Here's how the part is built. I have some questions about the finished solid (model axes, mm). Face numbers are marked on the shaded views. A direction names the side the tool comes from. Give positions to 0.01 mm unless a question says otherwise; leave off trailing zeros. Write each loop counter-clockwise with the first axis right and the second up, starting at its lowest first coordinate (ties: lowest second). Pieces come first, ordered by that corner, then holes. Notation, with made-up numbers: (-23, -20.5) - (-1, -20.5) arc R22 cw to (-1, 14.5) - close; hole circle Ø10 at (52.25, -20). An arc over 180 degrees is marked (long way). Write each question's results on one line, items separated by ' | '. Start each with the question number.
Item 1: Suppose I cut it at C-C on x = -283.5. List the corners of the cut face in (y, z) for me.
Item 2: Suppose I cut it at B-B on z = 50.8. List the corners of the cut face in (x, y) for me.
Item 3: Will these pins go through, and if not, where does the flat tip stop? P1, Ø2, axis at y = 34.5, z = -12, coming from the -X side; P2, Ø3, axis at x = -248.5, y = 87.5, coming from the +Z side.
Item 4: We'd pull the mould along Y, two halves only. Please class the marked faces 1, 2 and 3: +Y half, -Y half, draft (parallel to the pull), parting line (faces both ways), or undercut.
Item 5: Which directions (+Z, -Z, +X, -X, +Y, -Y) give clear straight access to the entire face, cutting with the end or side of a thin tool? Please do the marked faces 4, 5 and 6.
Item 6: Suppose I cut it at D-D on x = -39. List the corners of the cut face in (y, z) for me.
Item 7: Suppose I cut it at A-A on y = 12.7. List the corners of the cut face in (x, z) for me.
Item 8: Please list where these lines run through material, in increasing order: line 1 along Z through (x, y) = (-79, 12); line 2 along Y through (x, z) = (-150.5, 50.8); line 3 along X through (y, z) = (-36, -40.5).
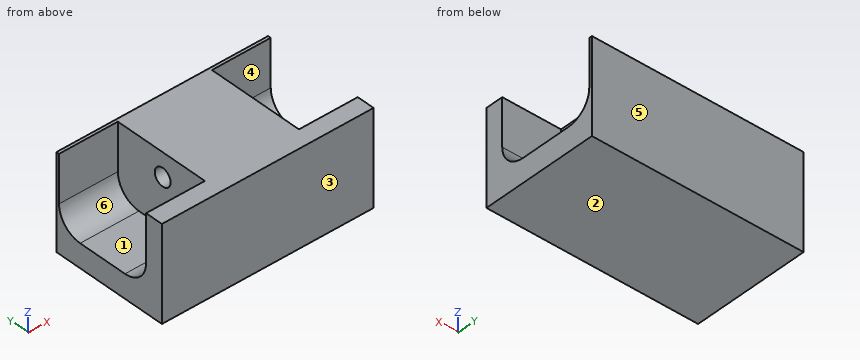
```python
from build123d import *

# Parameters (mm, degrees)
SKETCH1_W           = 203.2
SKETCH1_H           = 254
BOSS_EXTRUDE1_DEPTH = 114.3
CUT_EXTRUDE2_DEPTH  = 127
SKETCH3_R           = 19.05
CUT_EXTRUDE3_DEPTH  = 380.515441056


with BuildPart() as part:
    # Sketch1 → Boss-Extrude1 (new, symmetric)
    with BuildSketch(Plane(origin=(0, 0, 0), x_dir=(0, 0, -1), z_dir=(1, 0, 0))):
        Rectangle(SKETCH1_W, SKETCH1_H)
    extrude(amount=BOSS_EXTRUDE1_DEPTH, both=True)

    # Sketch2 → Cut-Extrude2 (cut)
    with BuildSketch(Plane(origin=(114.3, 0, 0), x_dir=(0, 0, -1), z_dir=(1, 0, 0))):
        with BuildLine():
            Line((-101.6, 120.65), (0, 120.65))
            ThreePointArc((0, 120.65), (35.921024484, 105.771024484), (50.8, 69.85))
            Line((50.8, 69.85), (50.8, -38.1))
            ThreePointArc((50.8, -38.1), (35.921024484, -74.021024484), (0, -88.9))
            Line((0, -88.9), (-101.6, -88.9))
            Line((-101.6, -88.9), (-101.6, 120.65))
        make_face()
    extrude(amount=-CUT_EXTRUDE2_DEPTH, mode=Mode.SUBTRACT)

    # Mirror1: part across plane


with BuildPart() as part_1:
    add(part.part)
    add(part.part.mirror(Plane(origin=(-114.3, 0, 0), x_dir=(0, 0, 1), z_dir=(1, 0, 0))))

    # Sketch3 → Cut-Extrude3 (cut, through all)
    with BuildSketch(Plane(origin=(0, 0, 0), x_dir=(0, 0, -1), z_dir=(1, 0, 0))):
        with Locations((-50.8, 12.7)):
            Circle(SKETCH3_R)
    extrude(amount=-CUT_EXTRUDE3_DEPTH, mode=Mode.SUBTRACT)


solid = part_1.part
```
Checked values:
1) outline: (-127, -101.6) - (127, -101.6) - (127, 101.6) - (120.65, 101.6) - (120.65, 0) arc R50.8 cw to (69.85, -50.8) - (-38.1, -50.8) arc R50.8 cw to (-88.9, 0) - (-88.9, 101.6) - (-127, 101.6) - close
2) outline: (-342.9, -127) - (114.3, -127) - (114.3, -88.9) - (-12.7, -88.9) - (-12.7, -6.35) - (-215.9, -6.35) - (-215.9, -88.9) - (-342.9, -88.9) - close; (-342.9, 120.65) - (-215.9, 120.65) - (-215.9, 31.75) - (-12.7, 31.75) - (-12.7, 120.65) - (114.3, 120.65) - (114.3, 127) - (-342.9, 127) - close
3) P1: stops at x = -215.9 | P2: stops at z = -47.05
4) face 1: undercut | face 2: draft | face 3: -Y half
5) face 4: +Z, +X | face 5: +Z, -Z, +X, -X, +Y | face 6: +Z, -X
6) outline: (-127, -101.6) - (127, -101.6) - (127, 101.6) - (-127, 101.6) - close; hole circle Ø38.1 at (12.7, 50.8)
7) outline: (-342.9, -101.6) - (114.3, -101.6) - (114.3, -50.8) - (-12.7, -50.8) - (-12.7, 31.75) - (-215.9, 31.75) - (-215.9, -50.8) - (-342.9, -50.8) - close; (-215.9, 69.85) - (-12.7, 69.85) - (-12.7, 101.6) - (-215.9, 101.6) - close
8) line 1: z = -101.6 to 31.76, 69.84 to 101.6 | line 2: y = -127 to -6.35, 31.75 to 127 | line 3: x = -215.9 to -12.7
